Build history of the part. All positions in model axes, mm. A direction names the side the tool comes from. Coordinates: 2 decimals unless noted, no trailing zeros. Order: outer loops, then holes, each group sorted by start corner. A loop starts at its lowest first (then second) coordinate and runs counter-clockwise, first axis right, second up. Notation, with made-up numbers: (-12.75, -24) - (44.25, -24) arc R6 cw to (44.25, -14) - close; hole circle Ø3 at (44.25, 26.25). An arc over 180 degrees is marked (long way). Return JSON: item names as keys, results as strings.
from build123d import *

# Parameters (mm, degrees)
F0_R     = 12.7
F1_DEPTH = 25.4
F4_R     = 12.7
F5_DEPTH = 25.4
F6_R     = 12.7


with BuildPart() as f1:
    # F0 (on Front) → F1 (new body)
    with BuildSketch(Plane.XZ):
        with BuildLine():
            Line((58.923879, -11.589798), (-30.463359, 37.426992))
            ThreePointArc((-30.463359, 37.426992), (-55.617447, 37.011684), (-68.076121, 15.155744))
            Line((-68.076121, 15.155744), (-68.076121, -35.644256))
            Line((-68.076121, -35.644256), (58.923879, -35.644256))
            Line((58.923879, -35.644256), (58.923879, -21.580534))
            Line((58.923879, -21.580534), (58.923879, -11.589798))
        make_face()
        with Locations((-42.676121, 15.155744)):
            Circle(F0_R, mode=Mode.SUBTRACT)
    extrude(amount=F1_DEPTH)

    # F4 (on face) → F5 (join)
    with BuildSketch(Plane.XZ.offset(25.4)):
        with BuildLine():
            Line((-17.407208, -18.995201), (-17.407208, 12.578534))
            ThreePointArc((-17.407208, 12.578534), (-20.191005, 26.970123), (-30.463359, 37.426992))
            ThreePointArc((-30.463359, 37.426992), (-55.617447, 37.011684), (-68.076121, 15.155744))
            Line((-68.076121, 15.155744), (-68.076121, -18.995201))
            Line((-68.076121, -18.995201), (-68.076121, -35.644256))
            Line((-68.076121, -35.644256), (58.923879, -35.644256))
            Line((58.923879, -35.644256), (58.923879, -18.995201))
            Line((58.923879, -18.995201), (-17.407208, -18.995201))
        make_face()
        with Locations((-42.676121, 15.155744)):
            Circle(F4_R, mode=Mode.SUBTRACT)
    extrude(amount=F5_DEPTH)

    # F6
    f6_edges = [f1.edges().sort_by_distance(p)[0] for p in [
        (58.923879, -50.8, -27.319728),
    ]]
    fillet(f6_edges, radius=F6_R)


solid = f1.part
1. Probe L1, parallel to Y at x = 14.5, z = 7; L2, parallel to X at y = -48.5, z = -5; L3, parallel to Z at x = 49.5, y = -46. List the from-to ranges inside material, lowest first.
Check values:
{"L1": "-25.4 to 0", "L2": "-68.08 to -17.41", "L3": "-35.64 to -19"}
2. Tool access for faces 4 (the flat face through (-24, -50.8, -5)), 5 (the flat face through (4, -25.4, -3)): list every direction of +Z, -Z, +X, -X, +Y, -Y with a clear straight run to the whole face (end or side of a thin tool).
Check values:
{"face 4": "+Z, -Z, +X, -X, -Y", "face 5": "+Z, +X, -Y"}
3. Drop flat-ended pins along their axis: pin 1 (1 mm diameter, centred on y = -45, z = -22, fed in from +X); pin 2 (1.5 mm diameter, centred on x = -13, z = -0.5, fed in from -Y); pin 3 (3 mm diameter, centred on y = -35.5, z = 32, fed in from -X). Give the stop position or say it passes through.
Check values:
{"pin 1": "x = 57.19", "pin 2": "y = -25.4", "pin 3": "x = -62.92"}
4. Cut at A-A on y = -32. Give the cut face in (x, z).
Check values:
{"outline": "(-68.08, -35.64) - (58.92, -35.64) - (58.92, -19) - (-17.41, -19) - (-17.41, 12.58) arc R25.4 ccw to (-30.46, 37.43) arc R25.4 ccw to (-68.08, 15.16) - close; hole circle Ø25.4 at (-42.68, 15.16)"}
5. Cut at C-C on z = 21. Give the cut face in (x, y).
Check values:
{"outline": "(-67.39, -50.8) - (-53.95, -50.8) - (-53.95, 0) - (-67.39, 0) - close; (-31.4, -50.8) - (-17.96, -50.8) - (-17.96, -25.4) - (-0.51, -25.4) - (-0.51, 0) - (-31.4, 0) - close"}
6. Mould opens along Z. For faces 1 (the flat face through (-17.407, -38, -3)), 2 (the flat face through (-68.076, -25, -10)), 3 (the flat face through (-5, -25, -35.644)) say: pulls with the +Z half, pulls with the -Z half, needs draft (parallel to the pull), parting line crosses it, or undercut.
Check values:
{"face 1": "undercut", "face 2": "needs draft", "face 3": "pulls with the -Z half"}
7. Cut at D-D on z = -4.5. Give the cut face in (x, y).
Check values:
{"outline": "(-68.08, -50.8) - (-17.41, -50.8) - (-17.41, -25.4) - (45.99, -25.4) - (45.99, 0) - (-68.08, 0) - close"}
8. Cut at B-B on x = -43. Give the cut face in (y, z), plus the area to 3 significant figures.
Check values:
{"outline": "(-50.8, -35.64) - (0, -35.64) - (0, 2.46) - (-50.8, 2.46) - close; (-50.8, 27.85) - (0, 27.85) - (0, 40.55) - (-50.8, 40.55) - close", "area": "2,580 mm²"}
